Verification items for the finished model (mm, model axes). Give positions to 0.01 mm unless a question says otherwise; leave off trailing zeros. Order: outer loops, then holes, each group sorted by start corner. A loop starts at its lowest first (then second) coordinate and runs counter-clockwise, first axis right, second up.
(1) Scan lines: L1, parallel to X at y = 38.5, z = 0.95; L2, parallel to Y at x = -61, z = 1.9; L3, parallel to X at y = -23.5, z = 0.65. Record each from-to range of solid material in increasing order.
(2) Gauge pin test, flat ends, axial feed: pin 1 (4 mm diameter, centred on x = 5, y = 20, fed in from -Z); pin 2 (1.4 mm diameter, centred on x = -61, y = 38.5, fed in from -Z). Record the tip position at first contact, or that the pin passes through.
(3) Sectioned sample at A-A on y = 23.5. Record the cut outline in (x, z), plus the area to 3 significant figures.
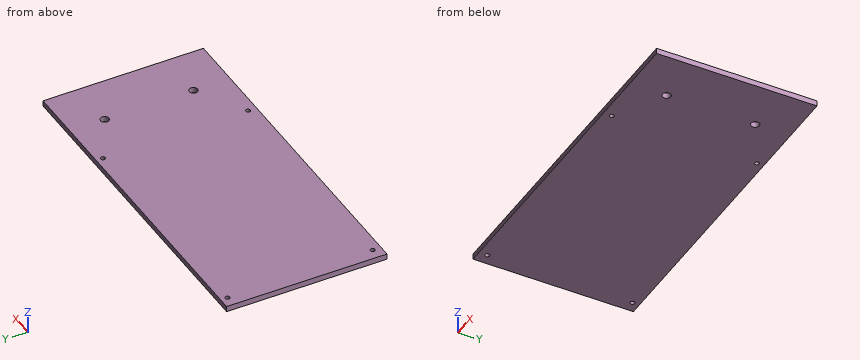
```python
from build123d import *

# Parameters (mm, degrees)
F0_W     = 180
F0_H     = 85
F1_DEPTH = 3
F2_D     = 2.4
F3_D     = 4.4


with BuildPart() as f1:
    # F0 (on Top) → F1 (new body)
    with BuildSketch(Plane.XY):
        with Locations((23.1652522087, -0.4566903412)):
            Rectangle(F0_W, F0_H)
    extrude(amount=F1_DEPTH)

    # F2 (through all)
    with Locations(Plane(origin=(0, 0, 0), x_dir=(1, 0, 0), z_dir=(0, 0, -1))):
        with Locations((-61, 38.5), (-61, -38.5), (61, 38.5), (61, -38.5)):
            Hole(F2_D / 2)

    # F3 (through all)
    with Locations(Plane(origin=(0, 0, 0), x_dir=(1, 0, 0), z_dir=(0, 0, -1))):
        with Locations((86.9170799851, -23.5), (86.9170799851, 23.5)):
            Hole(F3_D / 2)


solid = f1.part
```
Ans:
1. L1: x = -66.83 to -62.2, -59.8 to 59.8, 62.2 to 113.17
1. L2: y = -42.96 to -39.7, -37.3 to 37.3, 39.7 to 42.04
1. L3: x = -66.83 to 84.72, 89.12 to 113.17
2. pin 1: stops at z = 0
2. pin 2: passes through
3. outline: (-66.83, 0) - (84.72, 0) - (84.72, 3) - (-66.83, 3) - close; (89.12, 0) - (113.17, 0) - (113.17, 3) - (89.12, 3) - close
3. area: 527 mm2
